For this review, take the finished solid that the model builds, in its own axes (mm). A direction names the side the tool comes from. Coordinates: 2 decimals unless noted, no trailing zeros. Loops run counter-clockwise (first coordinate to the right, second up) from the corner with the lowest first, then second, coordinate; pieces in that order, holes last.
Autodesk Inventor part; units mm, degrees
ref_plane "YZ Plane" through (0, 0, 0) normal (1, 0, 0) x (0, 1, 0)
ref_plane "XZ Plane" through (0, 0, 0) normal (0, 1, 0) x (-1, 0, 0)
ref_plane "XY Plane" through (0, 0, 0) normal (0, 0, 1) x (1, 0, 0)
sketch "Эскиз1" plane through (0, 0, 0) normal (0, 0, 1) x (1, 0, 0)
  line L0 (0, 0) -> (-170, 0)
  line L1 (-170, 0) -> (-170, 10)
  line L2 (-170, 10) -> (0, 10)
  line L3 (0, 10) -> (0, 0)
  line L4 (-156.1916, 10) -> (-150.6349, 10) construction
  line L5 (-165, 10) -> (-158.1699, 3.1699)
  line L6 (-10, 10) -> (-34.5353, 10)
  line L7 (-30, 10) -> (-25, 10)
  line L8 (-23.8869, 10) -> (-18.8869, 10)
  line L9 (-15, 10) -> (-20, 10)
  line L10 (-170, 0) -> (-169, -1)
  line L11 (-170, 0) -> (-168.5858, 0) construction
  line L12 (-169, -1) -> (-169, 0)
  line L13 (-163.7026, 0) -> (-163.7026, -1)
  line L14 (-163.7026, -1) -> (-162.7026, 0)
  line L15 (0, 0) -> (-1, -1)
  line L16 (0, 0) -> (1.4142, 0) construction
  line L17 (-1, -1) -> (-1, 0)
  line L18 (-6, 0) -> (-6, -1)
  line L19 (-6, -1) -> (-7, 0)
  line L20 (-87, 0) -> (-87, -1)
  line L21 (-87, -1) -> (-88, 0)
  line L22 (-83, 0) -> (-83, -1)
  line L23 (-83, -1) -> (-82, 0)
  line L24 (-158.1699, 3.1699) -> (-160, 10)
  line L25 (-5, 10) -> (-11.8301, 3.1699)
  line L26 (-11.8301, 3.1699) -> (-10, 10)
  line L27 (-15, 10) -> (-21.8301, 3.1699)
  line L28 (-21.8301, 3.1699) -> (-20, 10)
  line L29 (-167.7026, 0) -> (-170, 2.2974)
  line L30 (-2, 0) -> (0, 2)
  point P0 (-170, 5)
  point P1 (-85, 0)
  point P2 (-161.5849, 6.5849)
  point P3 (-5, 10)
  point P4 (-15, 10)
  point P5 (-20, 10)
  dimension "d1" = 10
  dimension "d3" = 45
  dimension "d4" = 5
  dimension "d21" = 45
  dimension "d22" = 45
  dimension "d23" = 1
  dimension "d25" = 1
  dimension "d26" = 135
  dimension "d27" = 1
  dimension "d29" = 1
  dimension "d30" = 45
  dimension "d31" = 2
  dimension "d32" = 45
  dimension "d33" = 1
  dimension "d34" = 1
  dimension "d35" = 2
  dimension "d36" = 45
  dimension "d37" = 75
  dimension "d38" = 5
  dimension "d43" = 150
  dimension "d44" = 5
  dimension "d51" = 45
  dimension "d52" = 75
  dimension "d53" = 5
  dimension "d54" = 5
  dimension "d59" = 45
  dimension "d60" = 75
  dimension "d67" = 5
  dimension "d69" = 45
  dimension "d70" = 4
  dimension "d71" = 45
  dimension "d72" = 2
  dimension "d73" = 4
extrude "Выдавливание1" add sketch "Эскиз1" along normal blind 4 contours L30 L0 L29 L1 L2 L5 L24 L28 L27 L26 L25 L3 | L18 L19 L0 | L14 L13 L0
fillet "Сопряжение2" radius 1 2 edges at (0, 10, 2) (-170, 10, 2)
fillet "Сопряжение3" radius 1 8 edges at (-21.8301, 3.1699, 2) (-11.8301, 3.1699, 2) (-10, 10, 2) (-5, 10, 2) (-20, 10, 2) (-158.1699, 3.1699, 2) (-165, 10, 2) (-160, 10, 2)
properties part number "trunk 2"
Q1. Consider section B-B (x = -124). State the section outline as (y, z) points.
Q2. For pin 1 Ø0.5 at (y, z) = (-0.5, 2.5) entering from +X; pin 2 Ø2 at (x, z) = (-49, 2) entering from -Y; pin 3 Ø1 at (y, z) = (1, 0.5) entering from +X, all flat-tipped, find the tip position at first contact; note any pin that passes through.
Q3. The part is to be moulded in two halves that separate along X. For faces 4 (the face through (-86, 5, 4)), 5 (the face through (-170, 6, 2)), 6 (the face through (-7, 8, 2)), say which applies: +X half, -X half, draft (parallel to the pull), parting line (faces both ways), or undercut.
Q4. Machinability: for faces 1 (the face through (-4, 0, 2)), 2 (the face through (-17, 8, 2)), 3 (the face through (-166, 0, 2)), which of the approach directions +Z, -Z, +X, -X, +Y, -Y give a long, thin tool a straight path to every point of the face, cutting with its end or side? Answer none if there is none.
Q5. Wall thickness on probe 1 along X at (y, z) = (9.75, 2.65); probe 2 along X at (y, z) = (6, 3.15); probe 3 along Y at (x, z) = (-116.5, 3): over which ranges is each line inside the solid? List them lowest first.
Model answer:
1. outline: (0, 0) - (10, 0) - (10, 4) - (0, 4) - close
2. pin 1: stops at x = -6
2. pin 2: stops at y = 0
2. pin 3: stops at x = -0.5
3. face 4: draft
3. face 5: -X half
3. face 6: undercut
4. face 1: +Z, -Z, +X, -Y
4. face 2: +Z, -Z, +Y
4. face 3: +Z, -Z, -X, -Y
5. probe 1: x = -169.66 to -164.75, -159.36 to -20.64, -15.25 to -10.64, -5.25 to -0.34
5. probe 2: x = -170 to -161, -159.25 to -20.75, -19 to -10.75, -9 to 0
5. probe 3: y = 0 to 10
